Input: part model. Units: mm. Frame: model coordinates. Coordinates: 2 decimals unless noted, no trailing zeros. Order: outer loops, then holes, each group sorted by start corner. A loop starts at its lowest first (then second) coordinate and runs counter-clockwise, first axis right, second up. Notation, with made-up numbers: (26.5, 83) - (35.5, 83) arc R7 cw to (35.5, 91) - close; hole circle Ø4 at (-7, 28.25). An arc over 180 degrees is marked (long way). One line per question, with ' | ' between items.
from build123d import *

# Parameters (mm, degrees)
F0_R     = 127
F0_R_2   = 5
F1_DEPTH = 5
F2_DEPTH = 5
F3_SIZE2 = 4.662565
F3_SIZE  = 4.99999


# Not quite as in the source:
# - a fillet or chamfer is up to 0.001 mm smaller than in the source, because OpenCascade refuses the exact size


with BuildPart() as f1:
    # F0 (on Front) → F1 (new body, symmetric)
    with BuildSketch(Plane.XZ):
        Circle(F0_R)
        Circle(F0_R_2, mode=Mode.SUBTRACT)
    extrude(amount=F1_DEPTH, both=True)

    # F0 (on Front) → F2 (join, symmetric)
    with BuildSketch(Plane.XZ):
        Circle(F0_R_2)
    extrude(amount=F2_DEPTH, both=True)

    # F3 (size 5 and 4.6625754307 in the source; OpenCascade refuses exactly that, so slightly less here)
    f3_edges = [f1.edges().sort_by_distance(p)[0] for p in [
        (-127, 5, 0),
        (-127, -5, 0),
    ]]
    f3_side = f1.faces().sort_by_distance((-127, 0, 0))[0]
    chamfer(f3_edges, length=F3_SIZE, length2=F3_SIZE2, reference=f3_side)


solid = f1.part
Item 1: Contact query for flat-ended pins moving along their axis: P1, Ø2, axis at x = -96, y = -2.5, coming from the -Z side; P2, Ø1.5, axis at y = -2, z = -96.5, coming from the -X side. Output: stop coordinate, or through.
Data:
P1: z = -81.41 | P2: x = -81.08
Item 2: Ray query, line 1 (Z direction, x = -11, y = 1.5); line 2 (X direction, y = 4.5, z = 110.5); line 3 (Z direction, x = 115.5, y = -0.5). Return the intervals inside material, ascending.
Data:
line 1: -125.12 to 125.12 | line 2: -53.58 to 53.58 | line 3: -51.68 to 51.68
Item 3: Section C-C on y = -2. Return the cut outline in (x, z).
Data:
outline: circle Ø250.27 at (0, 0)
